```python
from build123d import *

# Parameters (mm, degrees)
SKETCH1_R           = 9.5
BOSS_EXTRUDE1_DEPTH = 1.52
SKETCH2_R           = 8.05
CUT_EXTRUDE1_DEPTH  = 2.52
CHAMFER1_SIZE       = 0.3


with BuildPart() as part:
    # Sketch1 → Boss-Extrude1 (new body)
    with BuildSketch(Plane(origin=(0, 0, 0), x_dir=(1, 0, 0), z_dir=(0, 1, 0))):
        Circle(SKETCH1_R)
    extrude(amount=BOSS_EXTRUDE1_DEPTH)

    # Sketch2 → Cut-Extrude1 (cut, through all)
    with BuildSketch(Plane(origin=(0, 1.52, 0), x_dir=(1, 0, 0), z_dir=(0, 1, 0))):
        Circle(SKETCH2_R)
    extrude(amount=-CUT_EXTRUDE1_DEPTH, mode=Mode.SUBTRACT)

    # Chamfer1
    chamfer1_edges = [part.edges().sort_by_distance(p)[0] for p in [
        (-8.05, 0, 0),
    ]]
    chamfer(chamfer1_edges, length=CHAMFER1_SIZE)


solid = part.part
```
Check sheet for the modelled part. Datum: model origin and axes. Units: mm. Give positions to 0.01 mm unless a question says otherwise; leave off trailing zeros. Write each loop counter-clockwise with the first axis right and the second up, starting at its lowest first coordinate (ties: lowest second). Pieces come first, ordered by that corner, then holes. Notation, with made-up numbers: (66, -23.5) -> (70, -23.5) arc R10 cw to (70, -19.5) -> close; hole circle Ø5 at (6, 44). An arc over 180 degrees is marked (long way). Use CSV: the item, a comma, the result in double quotes. Start each with the question number.
Q1. Scan lines: line 1 along X through (y, z) = (0.9, 0); line 2 along X through (y, z) = (0.15, -1). Record each from-to range of solid material in increasing order.
Q2. Depth check by flat-ended pin: P1, Ø10, axis at x = -5, z = -1, coming from the +Y side. Enter the tip coordinate at first touch or a pass-through.
Q3. Cross-section at A-A on z = 0. Enter the section's corners in (x, y), and give its area (3 significant figures).
Q4. Release check for a two-part mould opening along X. For faces 1 (the cylindrical face through (4.38, 0.75, 8.43)), 2 (the flat face through (-8, 1.52, -2)), 3 (the cylindrical face through (7.678, 0.919, -2.418)) record: +X half, -X half, draft (parallel to the pull), parting line (faces both ways), or undercut.
Q5. Cross-section at B-B on x = 0. Enter the section's corners in (y, z).
Working result:
1,line 1,"x = -9.5 to -8.05, 8.05 to 9.5"
1,line 2,"x = -9.45 to -8.14, 8.14 to 9.45"
2,P1,"stops at y = 1.52"
3,outline,"(-9.5, 0) -> (-8.35, 0) -> (-8.05, 0.3) -> (-8.05, 1.52) -> (-9.5, 1.52) -> close; (8.05, 0.3) -> (8.35, 0) -> (9.5, 0) -> (9.5, 1.52) -> (8.05, 1.52) -> close"
3,area,"4.32 mm^2"
4,face 1,"parting line"
4,face 2,"draft"
4,face 3,"undercut"
5,outline,"(0, -9.5) -> (1.52, -9.5) -> (1.52, -8.05) -> (0.3, -8.05) -> (0, -8.35) -> close; (0, 8.35) -> (0.3, 8.05) -> (1.52, 8.05) -> (1.52, 9.5) -> (0, 9.5) -> close"
